Design review of the part built by this model. Coordinates are the model's own, in mm. Coordinates: 2 decimals unless noted, no trailing zeros. Order: outer loops, then holes, each group sorted by start corner. A loop starts at its lowest first (then second) coordinate and runs counter-clockwise, first axis right, second up. Notation, with made-up numbers: (86, -31.5) -> (114, -31.5) arc R22 cw to (114, -21.5) -> close; hole circle Ø9 at (24, 56.25). An arc over 180 degrees is marked (long way). Write item = value, one per line.
```python
from build123d import *

# Parameters (mm, degrees)
F0_R     = 15.875
F1_DEPTH = 113.5126
F2_R     = 12.7
F3_DEPTH = 113.5126


# Not quite as in the source:
# - a fillet or chamfer that OpenCascade refuses, or shapes differently, is made with other operations: its cross-section is extruded or revolved along the edge and cut away or added


with BuildPart() as f1:
    # F0 (on Front) → F1 (new body)
    with BuildSketch(Plane.XZ):
        Circle(F0_R)
    extrude(amount=F1_DEPTH)

    # F2 (on face) → F3 (cut)
    with BuildSketch(Plane.XZ.offset(113.5126)):
        Circle(F2_R)
    extrude(amount=-F3_DEPTH, mode=Mode.SUBTRACT)

    # F4: fillet of radius 6.35 on 1 edges, made by hand

    # F4_s1 → F4_t2 (revolve, cut)
    with BuildSketch(Plane.XY):
        with BuildLine():
            ThreePointArc((15.875, -108.013338686), (15.024261314, -111.188338686), (12.7, -113.5126))
            Line((12.7, -113.5126), (15.875, -113.5126))
            Line((15.875, -113.5126), (15.875, -108.013338686))
        make_face()
    revolve(axis=Axis((0, -113.5126, 0), (0, -1, 0)), mode=Mode.SUBTRACT)

    # F5: fillet of radius 6.35 on 1 edges, made by hand

    # F5_s1 → F5_t2 (revolve, cut)
    with BuildSketch(Plane.XY):
        with BuildLine():
            ThreePointArc((15.875, -5.499261314), (15.024261314, -2.324261314), (12.7, 0))
            Line((12.7, 0), (15.875, 0))
            Line((15.875, 0), (15.875, -5.499261314))
        make_face()
    revolve(axis=Axis((0, 0, 0), (0, -1, 0)), mode=Mode.SUBTRACT)


solid = f1.part
```
(1) We need section B-B (z = 0). Write out the cut boundary in (x, y) (3 decimals), and give its area (3 significant figures).
Report:
outline = (-15.875, -108.013) arc R6.35 ccw to (-12.7, -113.513) -> (-12.7, 0) arc R6.35 ccw to (-15.875, -5.499) -> close; (12.7, -113.513) arc R6.35 ccw to (15.875, -108.013) -> (15.875, -5.499) arc R6.35 ccw to (12.7, 0) -> close
area = 700 mm²
(2) We need section C-C (y = -23.5). Write out the cut boundary in (x, z) (3 decimals).
Report:
outline = circle Ø31.75 at (0, 0); hole circle Ø25.4 at (0, 0)
(3) We need section A-A (x = 0). Write out the cut boundary in (y, z) (3 decimals).
Report:
outline = (-113.513, -12.7) arc R6.35 ccw to (-108.013, -15.875) -> (-5.499, -15.875) arc R6.35 ccw to (0, -12.7) -> close; (-113.513, 12.7) -> (0, 12.7) arc R6.35 ccw to (-5.499, 15.875) -> (-108.013, 15.875) arc R6.35 ccw to start
(4) For L1, parallel to Z at x = 0, y = -72 (3 decimals); L2, parallel to X at y = -18.5, z = -10; L3, parallel to Z at x = -3.5, y = -98, list the stretches that pass through material, from the lowest coordinate up.
Report:
L1 = -15.875 to -12.7, 12.7 to 15.875
L2 = -12.33 to -7.83, 7.83 to 12.33
L3 = -15.48 to -12.21, 12.21 to 15.48
(5) The part is to be moulded in two halves that separate along X. For faces 1 (the cylindrical face through (-3.441, -56.039, -15.497)), 2 (the cylindrical face through (-2.75, -57.55, -12.4)), say which applies: released by +X, released by -X, zero draft, split by the parting line, or undercut.
Report:
face_1 = split by the parting line
face_2 = undercut
(6) Insertion check: pin 1 (8 mm diameter, centred on x = -4.5, y = -48, fed in from -Z); pin 2 (3 mm diameter, centred on y = -79, z = -7, fed in from +X); pin 3 (8 mm diameter, centred on y = -87.5, z = 12, fed in from -X); pin 4 (6 mm diameter, centred on x = 9.5, z = -11.5, fed in from +Y). Each pin has a flat end and moves straight along its axis. Give the tip position at first contact, or say it passes through.
Report:
pin_1 = -15.87
pin_2 = 14.89
pin_3 = -13.71
pin_4 = 0
